Work out the finished part from the listing and answer in its coordinate system (mm). Face numbers are marked on the shaded views. A direction names the side the tool comes from. Coordinates: 2 decimals unless noted, no trailing zeros. Loops run counter-clockwise (first coordinate to the right, second up) from the corner with the lowest first, then second, coordinate; pieces in that order, holes last. Notation, with made-up numbers: (12.5, 41) -> (31.5, 41) arc R9 ccw to (31.5, 51) -> close; hole circle Ø6 at (42, -25.5). An arc over 180 degrees is marked (long way). Answer as CSV lines item,"result".
Solid Edge part; units mm, degrees
sketch "Sketch1" plane through (0, 0, 0) normal (1, 0, 0) x (0, 1, 0)
  line L0 (0, -1.6764) -> (0, 1.6764)
  arc A0 (0, 1.6764) -> (5.55625, -1.6764) centre (-0.25374, -5.024398) cw
  line L1 (0, -1.6764) -> (5.55625, -1.6764)
revolve "RevolvedProtrusion1" add sketch "Sketch1" angle 360 about axis through (0, 0, -14.779625) along (0, 0, 1)
sketch "Sketch2" plane through (0, 0, -1.6764) normal (0, 0, -1) x (0, 1, 0)
  circle A0 centre (0, 0) radius 3.175
extrude "Protrusion1" add sketch "Sketch2" along normal blind 50.8
sketch "Sketch3" plane through (0, 0, -52.4764) normal (0, 0, -1) x (1, 0, 0)
  circle A0 centre (0, 0) radius 3.17246
extrude "Cutout1" cut sketch "Sketch3" against normal blind 49.2125 flip side to cut
sketch "Sketch4" plane through (-0.603226, 0.360624, 3.3528) normal (0, 0, 1) x (1, 0, 0)
  line L0 (-0.542454, 1.623751) -> (1.748905, 1.623751)
  line L1 (2.894585, -0.360624) -> (1.748905, 1.623751)
  line L2 (1.748905, -2.344999) -> (2.894585, -0.360624)
  line L3 (-0.542454, -2.344999) -> (1.748905, -2.344999)
  line L4 (-1.688133, -0.360624) -> (-0.542454, -2.344999)
  line L5 (-0.542454, 1.623751) -> (-1.688133, -0.360624)
extrude "ExtrudedCutout_11" cut sketch "Sketch4" against normal blind 5.0292
properties part number "24100156"
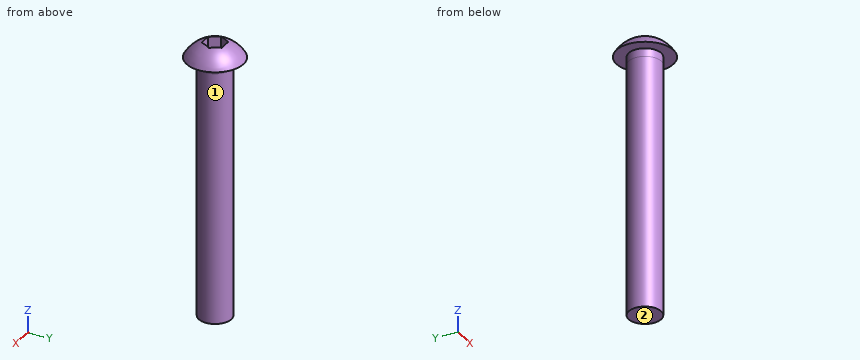
(1) Flat-ended cylindrical pins translate along their axes: pin 1 Ø1 at (x, y) = (3, -3.5) entering from -Z; pin 2 Ø1 at (x, y) = (1.5, 3) entering from +Z; pin 3 Ø2 at (y, z) = (1, -10) entering from +X; pin 4 Ø6 at (x, y) = (-3.5, 2.5) entering from +Z. Find the tip coordinate at first contact, or state that the pin passes through.
Computed values:
pin 1,"z = -1.68"
pin 2,"z = 0.92"
pin 3,"x = 3.17"
pin 4,"z = 1.3"
(2) Consider line 1 along X through (y, z) = (0.25, -27); line 2 along Y through (x, z) = (0, -10.5); line 3 along Z through (x, y) = (1.25, 0.75). Determine where each line is inside the solid, lowest interval first.
Computed values:
line 1,"-3.16 to 3.16"
line 2,"-3.17 to 3.17"
line 3,"-52.48 to -1.68"
(3) A cutting plane is placed at A-A, the plane z = -24. Write down the section's boundary in (x, y), and give its area (3 significant figures).
Computed values:
outline,"circle Ø6.34 at (0, 0)"
area,"31.6 mm2"
(4) Which of the six approach directions +Z, -Z, +X, -X, +Y, -Y give full straight-line access (tool end or side, diameter ignored) to the marked faces 1 and 2?
Computed values:
face 1,"-Z"
face 2,"-Z, +X, -X, +Y, -Y"
